Read the model definition and answer for the solid it produces. Units are mm, in the model's axes. A direction names the side the tool comes from. Coordinates: 2 decimals unless noted, no trailing zeros. Write each loop counter-clockwise with the first axis right and the second up, starting at its lowest first coordinate (ties: lowest second). Pieces come first, ordered by that corner, then holes. Notation, with made-up numbers: (79.25, 16) -> (116.25, 16) arc R26 ccw to (116.25, 46) -> close; hole circle Ø3 at (64.5, 24.25). An arc over 180 degrees is marked (long way). Answer as a JSON object with one key per item and string values. Group by question number.
(1) Straight lines are drawn through the part: L1, parallel to X at y = -4.75, z = 8; L2, parallel to Y at x = 2, z = 30.5; L3, parallel to X at y = -2, z = 28. For each, find the intervals that lie inside material, in ascending order.
(2) Find section C-C (x = 3.2). Give the vertices of the cut face in (y, z).
(3) Flat-ended cylindrical pins translate along their axes: P1, Ø2, axis at x = 2.5, z = 32, coming from the +Y side; P2, Ø1, axis at x = 5, z = 19, coming from the -Y side. Find the tip coordinate at first contact, or state that the pin passes through.
(4) Which of the six approach directions +Z, -Z, +X, -X, +Y, -Y give full straight-line access (tool end or side, diameter ignored) to faces 1 (the face through (4.7, -2, 23)), 2 (the face through (5, -3, 0))?
(5) For a pull along X with two mould halves and no side action, classify faces 3 (the face through (1.1, -2, 23)), 4 (the face through (5.8, -0.5, 22.7)), 5 (the face through (0, -0.6, 22.7)) as +X half, -X half, draft (parallel to the pull), parting line (faces both ways), or undercut.
(6) Find section A-A (y = -3). Give the vertices of the cut face in (x, z).
(7) Find section B-B (z = 9). Give the vertices of the cut face in (x, y).
from build123d import *

# Parameters (mm, degrees)
EXTRUSION1_DEPTH = 46


with BuildPart() as part:
    # Esquisse1 → Extrusion1 (new body)
    with BuildSketch(Plane.XY):
        with BuildLine():
            Line((4.7, -4.8), (4.7, 0))
            Line((4.7, 0), (5.8, 0))
            Line((5.8, 0), (5.8, -1.1))
            Line((5.8, -1.1), (5.25, -1.6))
            Line((5.25, -1.6), (5.8, -2.1))
            Line((5.8, -2.1), (5.8, -4.8))
            ThreePointArc((5.8, -4.8), (5.33137085, -5.93137085), (4.2, -6.4))
            Line((4.2, -6.4), (1.6, -6.4))
            ThreePointArc((1.6, -6.4), (0.46862915, -5.93137085), (0, -4.8))
            Line((0, -4.8), (0, -2.1))
            Line((0, -2.1), (0.55, -1.6))
            Line((0.55, -1.6), (0, -1.1))
            Line((0, -1.1), (0, 0))
            Line((0, 0), (1.1, 0))
            Line((1.1, 0), (1.1, -4.8))
            ThreePointArc((1.1, -4.8), (1.246446609, -5.153553391), (1.6, -5.3))
            Line((1.6, -5.3), (4.2, -5.3))
            ThreePointArc((4.2, -5.3), (4.553553391, -5.153553391), (4.7, -4.8))
        make_face()
    extrude(amount=EXTRUSION1_DEPTH)


solid = part.part
Results below:
{
 "1": {"L1": "x = 0 to 1.1, 4.7 to 5.8", "L2": "y = -6.4 to -5.3", "L3": "x = 0.11 to 1.1, 4.7 to 5.69"},
 "2": {"outline": "(-6.4, 0) -> (-5.3, 0) -> (-5.3, 46) -> (-6.4, 46) -> close"},
 "3": {"P1": "stops at y = -5.29", "P2": "stops at y = -6.37"},
 "4": {"face 1": "+Z, -Z, +Y", "face 2": "-Z, +X, -X, +Y, -Y"},
 "5": {"face 3": "undercut", "face 4": "+X half", "face 5": "-X half"},
 "6": {"outline": "(0, 0) -> (1.1, 0) -> (1.1, 46) -> (0, 46) -> close; (4.7, 0) -> (5.8, 0) -> (5.8, 46) -> (4.7, 46) -> close"},
 "7": {"outline": "(0, -4.8) arc R1.6 ccw to (1.6, -6.4) -> (4.2, -6.4) arc R1.6 ccw to (5.8, -4.8) -> (5.8, -2.1) -> (5.25, -1.6) -> (5.8, -1.1) -> (5.8, 0) -> (4.7, 0) -> (4.7, -4.8) arc R0.5 cw to (4.2, -5.3) -> (1.6, -5.3) arc R0.5 cw to (1.1, -4.8) -> (1.1, 0) -> (0, 0) -> (0, -1.1) -> (0.55, -1.6) -> (0, -2.1) -> close"}
}
